Can you work these out from the model? Positions are in its coordinate system, mm. Face numbers are marked on the shaded views. A direction names the side the tool comes from. Coordinates: 2 decimals unless noted, no trailing zeros. Write each loop counter-clockwise with the first axis right and the second up, starting at its lowest first coordinate (ties: lowest second). Pieces come first, ordered by that corner, then holes. Notation, with made-up numbers: (9, 22.25) -> (24, 22.25) arc R26 cw to (24, 36.25) -> close; hole circle Ø8 at (-36, 39). An arc over 180 degrees is marked (long way). Use one line per item in the form item = value.
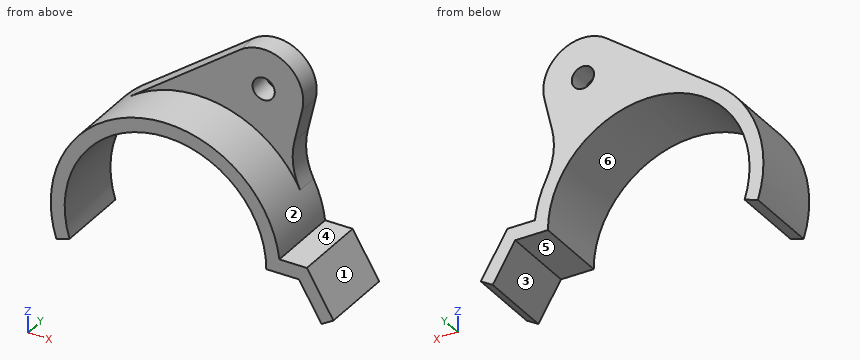
```python
from build123d import *

# Parameters (mm, degrees)
BOSS_EXTRUDE1_DEPTH = 109
BOSS_EXTRUDE2_DEPTH = 32
FILLET1_R           = 100
SKETCH4_R           = 16
CUT_EXTRUDE1_DEPTH  = 32


with BuildPart() as part:
    # Sketch2 → Boss-Extrude1 (new body)
    with BuildSketch(Plane(origin=(0, 0, 0), x_dir=(1, 0, 0), z_dir=(0, 1, 0))):
        with BuildLine():
            Line((0, 0), (47, 0))
            Line((47, 0), (79.447398719, 54.001539944))
            Line((79.447398719, 54.001539944), (96.590744733, 43.700778446))
            Line((96.590744733, 43.700778446), (58.315455564, -20))
            Line((58.315455564, -20), (18.783393542, -20))
            ThreePointArc((18.783393542, -20), (-180.560657841, -161.122436718), (-301.98658219, 50.79579719))
            Line((-301.98658219, 50.79579719), (-282.957905561, 44.638730864))
            ThreePointArc((-282.957905561, 44.638730864), (-167.595394372, -143.228656885), (0, 0))
        make_face()
    extrude(amount=-BOSS_EXTRUDE1_DEPTH)

    # Sketch3 → Boss-Extrude2 (add)
    with BuildSketch(Plane(origin=(0, 0, 0), x_dir=(1, 0, 0), z_dir=(0, 1, 0))):
        with BuildLine():
            Line((-242.764114638, -132.917936671), (-84.068153885, -249.642364452))
            ThreePointArc((-84.068153885, -249.642364452), (-18.943420898, -251.328541106), (5.227532222, -190.83193737))
            Line((5.227532222, -190.83193737), (-15.378785599, -102.094763712))
            ThreePointArc((-15.378785599, -102.094763712), (-122.836162355, -163.504630824), (-242.764114638, -132.917936671))
        make_face()
    extrude(amount=-BOSS_EXTRUDE2_DEPTH)

    # Fillet1
    fillet1_edges = [part.edges().sort_by_distance(p)[0] for p in [
        (-15.378785599, -16, 102.094763712),
    ]]
    fillet(fillet1_edges, radius=FILLET1_R)

    # Sketch4 → Cut-Extrude1 (cut)
    with BuildSketch(Plane(origin=(0, 0, 0), x_dir=(1, 0, 0), z_dir=(0, 1, 0))):
        with Locations(Location((-50.295096101, -203.725259056, 0), (0, 0, 270))):
            Circle(SKETCH4_R)
    extrude(amount=-CUT_EXTRUDE1_DEPTH, mode=Mode.SUBTRACT)


solid = part.part
```
Q1. Thinking about a two-plate mould opening in Z: for the marked faces 4, 5 and 6, which applies, released by +Z, released by -Z, zero draft, split by the parting line, or undercut?
Return value:
face_4 = released by +Z
face_5 = released by -Z
face_6 = undercut
Q2. Suppose I cut it at C-C (x = -145). Write out the boundary of the cut face in (y, z).
Return value:
outline = (-109, 145) -> (0, 145) -> (0, 204.83) -> (-32, 204.83) -> (-32, 165) -> (-109, 165) -> close
Q3. Will these pins go through, and if not, where does the flat tip stop? pin 1 (1 mm diameter, centred on y = -40, z = 42.5, fed in from -X); pin 2 (12 mm diameter, centred on x = -184, y = -96, fed in from -Z); pin 3 (12 mm diameter, centred on x = -23, y = -66, fed in from -Z).
Return value:
pin_1 = -304.57
pin_2 = 137.84
pin_3 = 68.12
Q4. If I drill on line 1 (Z direction, x = -145, y = -85); line 2 (Y direction, x = -65, z = 177); line 3 (X direction, y = -22, z = -38.5), over which ranges is the centre line in solid material (lowest first)? Write a range as from..to.
Return value:
line_1 = 145..165
line_2 = -32..0
line_3 = -305.45..-284.8, 70.13..93.47
Q5. Suppose I cut it at A-A (z = 33.5). Write out the boundary of the cut face in (x, y), then the cut area to 3 significant figures.
Return value:
outline = (-306.56, -109) -> (-286.08, -109) -> (-286.08, 0) -> (-306.56, 0) -> close; (-3.92, -109) -> (16.56, -109) -> (16.56, 0) -> (-3.92, 0) -> close
area = 4,470 mm2
Q6. Suppose I cut it at D-D (z = -21). Write out the boundary of the cut face in (x, y), then the cut area to 3 significant figures.
Return value:
outline = (-308.66, -109) -> (-288.47, -109) -> (-288.47, 0) -> (-308.66, 0) -> close; (59.62, -109) -> (82.95, -109) -> (82.95, 0) -> (59.62, 0) -> close
area = 4,740 mm2
Q7. Suppose I cut it at B-B (y = -42.5). Write out the boundary of the cut face in (x, z).
Return value:
outline = (-301.99, -50.8) -> (-282.96, -44.64) arc R145 cw (long way) to (0, 0) -> (47, 0) -> (79.45, -54) -> (96.59, -43.7) -> (58.32, 20) -> (18.78, 20) arc R165 ccw (long way) to start
Q8. For the marked faces 1, 2 and 3, which set-ups out of +Z, -Z, +X, -X, +Y, -Y let a thin tool reach every point of the face, with its end or its side?
Return value:
face_1 = +Z, +X, +Y, -Y
face_2 = -Y
face_3 = -Z, +Y, -Y
